The model under review builds one solid part; all positions refer to its coordinate system, in mm. Face numbers are marked on the shaded views. A direction names the side the tool comes from. Give positions to 0.01 mm unless a question says otherwise; leave off trailing zeros. Loops run counter-clockwise (first coordinate to the right, second up) from the corner with the lowest first, then second, coordinate; pieces in that order, holes last. Notation, with made-up numbers: (49, 58.5) -> (66, 58.5) arc R17 cw to (66, 72.5) -> close; hole circle Ø3 at (88.25, 40.25). An arc over 180 degrees is marked (long way). Write each question's results on one line, items separated by ' | '. Start each with the question number.
Q1. We need section A-A (z = 12.5). Give the number of separate pieces and of enclosed holes in the cut face, plus the area to 3 significant figures.
Q2. We need section D-D (y = 0). Write out the cut boundary in (x, z).
Q3. Machinability: for the marked faces 3, 4 and 5, which of the approach directions +Z, -Z, +X, -X, +Y, -Y give a long, thin tool a straight path to every point of the face, cutting with its end or side? Answer none if there is none.
Q4. We need section B-B (x = 0). Write out the cut boundary in (y, z).
Q5. Insertion check: pin 1 Ø3 at (y, z) = (15.5, 4) entering from +X; pin 2 Ø5 at (y, z) = (-20.5, 2.5) entering from +X; pin 3 Ø8 at (y, z) = (-18.5, -1.5) entering from -X. Each pin has a flat end and moves straight along its axis. Give the tip position at first contact, or say it passes through.
Q6. Wall thickness on L1, parallel to Y at x = 0, z = -1.5; L2, parallel to X at y = 0, z = 0.15; L3, parallel to Y at x = 20, z = 8: over which ranges is each line inside the solid? List them lowest first. Write a range as [from, to].
Q7. Mouldability with a two-part tool opening along X and no side actions: class the marked faces 1 and 2 as released by +X, released by -X, zero draft, split by the parting line, or undercut.
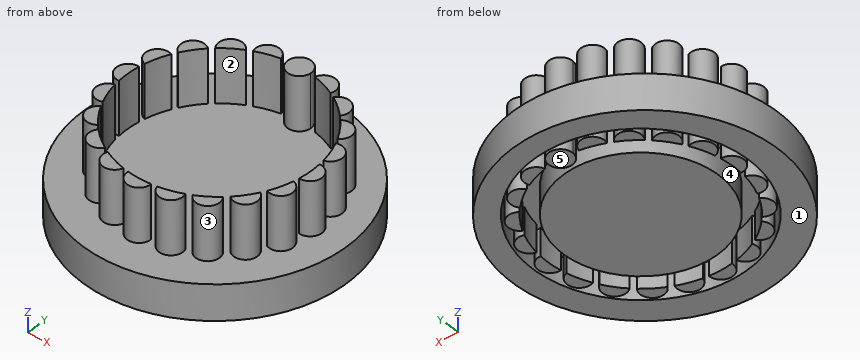
from build123d import *

# Parameters (mm, degrees)
EXTRUDE_1_DEPTH      = 3.710930537
EXTRUDE_1_DEPTH_BACK = 3.473333137
SKETCH_1_R           = 26.605035468
SKETCH_4_W           = 6.02260113
SKETCH_4_H           = 5.98653765
EXTRUDE_2_DEPTH      = 18


with BuildPart() as part:
    # 草图1 → 凸台-拉伸1 (new, two sides: drawn at the far end of the back side and taken through both)
    with BuildSketch(Plane(origin=(4.976775399, -23.162053726, 0), x_dir=(1, 0, 0), z_dir=(0, 0, 1)).offset(-EXTRUDE_1_DEPTH_BACK)):
        with Locations((-5.271905078, 22.51796653)):
            Circle(SKETCH_1_R)
    extrude(amount=EXTRUDE_1_DEPTH + EXTRUDE_1_DEPTH_BACK)

    # 草图4 → 切除-旋转1 (revolve, cut)
    with BuildSketch(Plane(origin=(0, 0, -0.114580032), x_dir=(1, 0, 0), z_dir=(0, 1, 0))):
        with Locations((-18.633409167, 0.825025845)):
            Rectangle(SKETCH_4_W, SKETCH_4_H)
    revolve(axis=Axis((0, 0, -21.724133591), (0, 0, 1)), mode=Mode.SUBTRACT)

    # 草图6 → 凸台-拉伸2 (add)
    with BuildSketch(Plane(origin=(0, 0, -3.473333137), x_dir=(-1, 0, 0), z_dir=(0, 0, -1))):
        with BuildLine():
            ThreePointArc((2.38482577, 18.602889633), (0, 21.144809988), (-2.38482577, 18.602889633))
            ThreePointArc((-2.38482577, 18.602889633), (0, 16.365449762), (2.38482577, 18.602889633))
        make_face()
        with BuildLine():
            ThreePointArc((-8.016713129, 16.955447716), (-5.795653863, 17.837188482), (-3.480504953, 18.429351099))
            ThreePointArc((-3.480504953, 18.429351099), (-6.534105629, 20.109909325), (-8.016713129, 16.955447716))
        make_face()
        with BuildLine():
            ThreePointArc((8.016713129, 16.955447716), (6.534105629, 20.109909325), (3.480504953, 18.429351099))
            ThreePointArc((3.480504953, 18.429351099), (5.795653863, 17.837188482), (8.016713129, 16.955447716))
        make_face()
        with BuildLine():
            ThreePointArc((-12.863868752, 13.648288441), (-11.023988745, 15.173218801), (-9.0051396, 16.451819274))
            ThreePointArc((-9.0051396, 16.451819274), (-12.428607474, 17.106510623), (-12.863868752, 13.648288441))
        make_face()
        with BuildLine():
            ThreePointArc((12.863868752, 13.648288441), (12.428607474, 17.106510623), (9.0051396, 16.451819274))
            ThreePointArc((9.0051396, 16.451819274), (11.023988745, 15.173218801), (12.863868752, 13.648288441))
        make_face()
        with BuildLine():
            ThreePointArc((-16.451819274, 9.0051396), (-15.173218801, 11.023988745), (-13.648288441, 12.863868752))
            ThreePointArc((-13.648288441, 12.863868752), (-17.106510623, 12.428607474), (-16.451819274, 9.0051396))
        make_face()
        with BuildLine():
            ThreePointArc((16.451819274, 9.0051396), (17.106510623, 12.428607474), (13.648288441, 12.863868752))
            ThreePointArc((13.648288441, 12.863868752), (15.173218801, 11.023988745), (16.451819274, 9.0051396))
        make_face()
        with BuildLine():
            ThreePointArc((-18.429351099, 3.480504953), (-17.837188482, 5.795653863), (-16.955447716, 8.016713129))
            ThreePointArc((-16.955447716, 8.016713129), (-20.109909325, 6.534105629), (-18.429351099, 3.480504953))
        make_face()
        with BuildLine():
            ThreePointArc((18.429351099, 3.480504953), (20.109909325, 6.534105629), (16.955447716, 8.016713129))
            ThreePointArc((16.955447716, 8.016713129), (17.837188482, 5.795653863), (18.429351099, 3.480504953))
        make_face()
        with BuildLine():
            ThreePointArc((-18.602889633, -2.38482577), (-18.755129875, 0), (-18.602889633, 2.38482577))
            ThreePointArc((-18.602889633, 2.38482577), (-21.144809988, 0), (-18.602889633, -2.38482577))
        make_face()
        with BuildLine():
            ThreePointArc((18.602889633, -2.38482577), (21.144809988, 0), (18.602889633, 2.38482577))
            ThreePointArc((18.602889633, 2.38482577), (18.755129875, 0), (18.602889633, -2.38482577))
        make_face()
        with BuildLine():
            ThreePointArc((-16.955447716, -8.016713129), (-17.837188482, -5.795653863), (-18.429351099, -3.480504953))
            ThreePointArc((-18.429351099, -3.480504953), (-20.109909325, -6.534105629), (-16.955447716, -8.016713129))
        make_face()
        with BuildLine():
            ThreePointArc((16.955447716, -8.016713129), (20.109909325, -6.534105629), (18.429351099, -3.480504953))
            ThreePointArc((18.429351099, -3.480504953), (17.837188482, -5.795653863), (16.955447716, -8.016713129))
        make_face()
        with BuildLine():
            ThreePointArc((-13.648288441, -12.863868752), (-15.173218801, -11.023988745), (-16.451819274, -9.0051396))
            ThreePointArc((-16.451819274, -9.0051396), (-17.106510623, -12.428607474), (-13.648288441, -12.863868752))
        make_face()
        with BuildLine():
            ThreePointArc((13.648288441, -12.863868752), (17.106510623, -12.428607474), (16.451819274, -9.0051396))
            ThreePointArc((16.451819274, -9.0051396), (15.173218801, -11.023988745), (13.648288441, -12.863868752))
        make_face()
        with BuildLine():
            ThreePointArc((-9.0051396, -16.451819274), (-11.023988745, -15.173218801), (-12.863868752, -13.648288441))
            ThreePointArc((-12.863868752, -13.648288441), (-12.428607474, -17.106510623), (-9.0051396, -16.451819274))
        make_face()
        with BuildLine():
            ThreePointArc((9.0051396, -16.451819274), (12.428607474, -17.106510623), (12.863868752, -13.648288441))
            ThreePointArc((12.863868752, -13.648288441), (11.023988745, -15.173218801), (9.0051396, -16.451819274))
        make_face()
        with BuildLine():
            ThreePointArc((-3.480504953, -18.429351099), (-5.795653863, -17.837188482), (-8.016713129, -16.955447716))
            ThreePointArc((-8.016713129, -16.955447716), (-6.534105629, -20.109909325), (-3.480504953, -18.429351099))
        make_face()
        with BuildLine():
            ThreePointArc((3.480504953, -18.429351099), (6.534105629, -20.109909325), (8.016713129, -16.955447716))
            ThreePointArc((8.016713129, -16.955447716), (5.795653863, -17.837188482), (3.480504953, -18.429351099))
        make_face()
        with BuildLine():
            ThreePointArc((2.38482577, -18.602889633), (0, -18.755129875), (-2.38482577, -18.602889633))
            ThreePointArc((-2.38482577, -18.602889633), (0, -21.144809988), (2.38482577, -18.602889633))
        make_face()
    extrude(amount=-EXTRUDE_2_DEPTH)


solid = part.part
Output:
1) separate pieces: 20 | enclosed holes: 0 | area: 193 mm2
2) outline: (-26.89, -3.47) -> (-21.64, -3.47) -> (-21.64, 2.05) -> (-21.14, 2.05) -> (-21.14, -3.47) -> (-18.76, -3.47) -> (-18.76, 2.05) -> (-15.62, 2.05) -> (-15.62, -3.47) -> (15.62, -3.47) -> (15.62, 2.05) -> (18.76, 2.05) -> (18.76, -3.47) -> (21.14, -3.47) -> (21.14, 2.05) -> (21.64, 2.05) -> (21.64, -3.47) -> (26.3, -3.47) -> (26.3, 3.71) -> (21.14, 3.71) -> (21.14, 14.53) -> (18.76, 14.53) -> (18.76, 3.71) -> (-18.76, 3.71) -> (-18.76, 14.53) -> (-21.14, 14.53) -> (-21.14, 3.71) -> (-26.89, 3.71) -> close
3) face 3: +Z | face 4: -Z | face 5: -Z, +X, -X, +Y, -Y
4) outline: (-27.25, -3.47) -> (-21.64, -3.47) -> (-21.64, 2.05) -> (-21.14, 2.05) -> (-21.14, -3.47) -> (-18.76, -3.47) -> (-18.76, 2.05) -> (-15.62, 2.05) -> (-15.62, -3.47) -> (15.62, -3.47) -> (15.62, 2.05) -> (16.37, 2.05) -> (16.37, -3.47) -> (21.14, -3.47) -> (21.14, 2.05) -> (21.64, 2.05) -> (21.64, -3.47) -> (25.96, -3.47) -> (25.96, 3.71) -> (21.14, 3.71) -> (21.14, 14.53) -> (16.37, 14.53) -> (16.37, 3.71) -> (-18.76, 3.71) -> (-18.76, 14.53) -> (-21.14, 14.53) -> (-21.14, 3.71) -> (-27.25, 3.71) -> close
5) pin 1: x = 21.9 | pin 2: x = 19.87 | pin 3: x = -23.01
6) L1: [-27.25, -21.64], [-21.14, -18.76], [-15.62, 15.62], [16.37, 21.14], [21.64, 25.96] | L2: [-26.89, -21.64], [-21.14, -18.76], [-15.62, 15.62], [18.76, 21.14], [21.64, 26.3] | L3: [-6.81, -4.78], [-2.04, 2.04], [4.78, 6.81]
7) face 1: zero draft | face 2: undercut
